```python
from build123d import *

# Parameters (mm, degrees)
SKETCH1_R           = 30
BOSS_EXTRUDE1_DEPTH = 4
SKETCH2_R           = 15
BOSS_EXTRUDE2_DEPTH = 10
SKETCH3_R           = 3
BOSS_EXTRUDE3_DEPTH = 4
SKETCH4_R           = 2
CUT_EXTRUDE1_DEPTH  = 4


with BuildPart() as part:
    # Sketch1 → Boss-Extrude1 (new body)
    with BuildSketch(Plane(origin=(0, 0, 0), x_dir=(1, 0, 0), z_dir=(0, 1, 0))):
        with Locations(Location((0, 0, 0), (0, 0, 270))):
            Circle(SKETCH1_R)
    extrude(amount=BOSS_EXTRUDE1_DEPTH)

    # Sketch2 → Boss-Extrude2 (add)
    with BuildSketch(Plane(origin=(0, 4, 0), x_dir=(1, 0, 0), z_dir=(0, 1, 0))):
        with Locations(Location((0, 0, 0), (0, 0, 270))):
            Circle(SKETCH2_R)
    extrude(amount=BOSS_EXTRUDE2_DEPTH)

    # Sketch3 → Boss-Extrude3 (add)
    with BuildSketch(Plane.XZ):
        with Locations(Location((-21, 0, 0), (0, 0, 90))):
            Circle(SKETCH3_R)
        with Locations(Location((0, 21, 0), (0, 0, 90))):
            Circle(SKETCH3_R)
        with Locations(Location((21, 0, 0), (0, 0, 90))):
            Circle(SKETCH3_R)
        with Locations(Location((0, -21, 0), (0, 0, 90))):
            Circle(SKETCH3_R)
    extrude(amount=BOSS_EXTRUDE3_DEPTH)

    # Sketch4 → Cut-Extrude1 (cut)
    with BuildSketch(Plane(origin=(0, 14, 0), x_dir=(1, 0, 0), z_dir=(0, 1, 0))):
        with Locations(Location((-5, 5, 0), (0, 0, 270))):
            Circle(SKETCH4_R)
        with Locations(Location((5, 5, 0), (0, 0, 270))):
            Circle(SKETCH4_R)
        with Locations(Location((5, -5, 0), (0, 0, 270))):
            Circle(SKETCH4_R)
        with Locations(Location((-5, -5, 0), (0, 0, 270))):
            Circle(SKETCH4_R)
    extrude(amount=-CUT_EXTRUDE1_DEPTH, mode=Mode.SUBTRACT)


solid = part.part
```
Read the model definition and answer for the solid it produces. Units are mm, in the model's axes. A direction names the side the tool comes from. Give positions to 0.01 mm unless a question says otherwise; leave off trailing zeros. Write each loop counter-clockwise with the first axis right and the second up, starting at its lowest first coordinate (ties: lowest second). Pieces come first, ordered by that corner, then holes. Notation, with made-up numbers: (25, 18.5) - (73, 18.5) arc R16 cw to (73, 39.5) - close; hole circle Ø2 at (87, 31). An arc over 180 degrees is marked (long way). Write item = value, one per line. Start each with the question number.
Item 1: Find section B-B (z = -19). Give the vertices of the cut face in (x, y).
Item 2: Each of these flat-tipped pins is pushed along its axis until it touches: P1, Ø5, axis at x = 5, z = 5, coming from the -Y side; P2, Ø8, axis at y = 1.5, z = -17.5, coming from the +X side; P3, Ø2, axis at x = -23.5, y = 0, coming from the -Z side; P4, Ø3, axis at x = 4, z = -5.5, coming from the +Y side. Where does it stop, or does it pass through?
Item 3: The mould has two halves that part along Z. Classify faces 4 (the cylindrical face through (1.32, 1.97, -29.97)), 5 (the flat face through (0, 14, 0)), 6 (the flat face through (-5, 10, 5)), 7 (the flat face through (5, 10, -5)): +Z half, -Z half, draft (parallel to the pull), parting line (faces both ways), or undercut.
Item 4: A tool of negligible diameter and unlimited length cuts with its end or side. For faces 1 (the cylindrical face through (0.66, 8.93, -14.985)), 2 (the flat face through (21, -4, 0)), 3 (the flat face through (0, 0, 0)), from which of +Z, -Z, +X, -X, +Y, -Y can it reach the whole face along a straight path? Write none if from no direction.
Item 5: Find section C-C (y = 5.75). Give the vertices of the cut face in (x, z).
Item 6: Find section D-D (x = -14). Give the vertices of the cut face in (y, z).
Item 7: Find the intervals of material crossed by probe 1 along X at (y, z) = (12.5, -5); probe 2 along Y at (x, z) = (-11.5, -4.5); probe 3 along Y at (x, z) = (22, 1.5), in increasing order. Write a range as [from, to].
Item 8: Find section A-A (x = 0). Give the vertices of the cut face in (y, z), then the cut area to 3 significant figures.
Response:
q1.outline = (-23.22, 0) - (-2.24, 0) - (-2.24, -4) - (2.24, -4) - (2.24, 0) - (23.22, 0) - (23.22, 4) - (-23.22, 4) - close
q2.P1 = 0
q2.P2 = 26.79
q2.P3 = -19.84
q2.P4 = 14
q3.face_4 = parting line
q3.face_5 = draft
q3.face_6 = undercut
q3.face_7 = undercut
q4.face_1 = +Y
q4.face_2 = +Z, -Z, +X, -X, -Y
q4.face_3 = -Y
q5.outline = circle Ø30 at (0, 0)
q6.outline = (0, -26.53) - (4, -26.53) - (4, -5.39) - (14, -5.39) - (14, 5.39) - (4, 5.39) - (4, 26.53) - (0, 26.53) - close
q7.probe_1 = [-14.14, -7], [-3, 3], [7, 14.14]
q7.probe_2 = [0, 14]
q7.probe_3 = [-4, 4]
q8.outline = (-4, -24) - (0, -24) - (0, -30) - (4, -30) - (4, -15) - (14, -15) - (14, 15) - (4, 15) - (4, 30) - (0, 30) - (0, 24) - (-4, 24) - (-4, 18) - (0, 18) - (0, -18) - (-4, -18) - close
q8.area = 588 mm²
